The drawing under review shows one solid part. Ordinate dimensions are in mm from its lowest x, y, z. A direction names the side the tool comes from. Give positions to 0.01 mm unless a question says otherwise; leave off trailing zeros. Order: outer loops, then holes, each group sorted by start corner. A loop starts at its lowest first (then second) coordinate and runs counter-clockwise, first axis right, second up. Notation, with made-up numbers: (43, -33) -> (47, -33) arc R27 ccw to (47, 2) -> close; hole circle Ø3 at (-7, -5). An arc over 180 degrees is marked (long way). Return JSON: item names as keys, results as strings. Group by question number.
1) To check wall thickness, follow line 1 along Z through (x, y) = (31.75, 20.85); line 2 along Y through (x, z) = (27, 4.5); line 3 along X through (y, z) = (24.25, 3). State the ranges of each line that lie inside material, in increasing order.
2) For the marked faces 1, 2, 3 and 4, list the 3-axis set-ups (+Z, -Z, +X, -X, +Y, -Y) from which the entire face can be reached by the end or side of a thin tool; tool diameter is ignored.
3) Add section C-C (x = 66.5). Give the boundary of the cut face in (y, z).
4) Add section A-A (x = 133.35). Give the boundary of the cut face in (y, z), then the cut area to 3 significant figures.
5) Insertion check: P1, Ø3, axis at y = 9.525, z = 6.35, coming from the +X side; P2, Ø5, axis at x = 31.75, z = 6.35, coming from the -Y side; P3, Ø4, axis at y = 24, z = 7.5, coming from the -X side. Each pin has a flat end and moves straight along its axis. Give the tip position at first contact, or say it passes through.
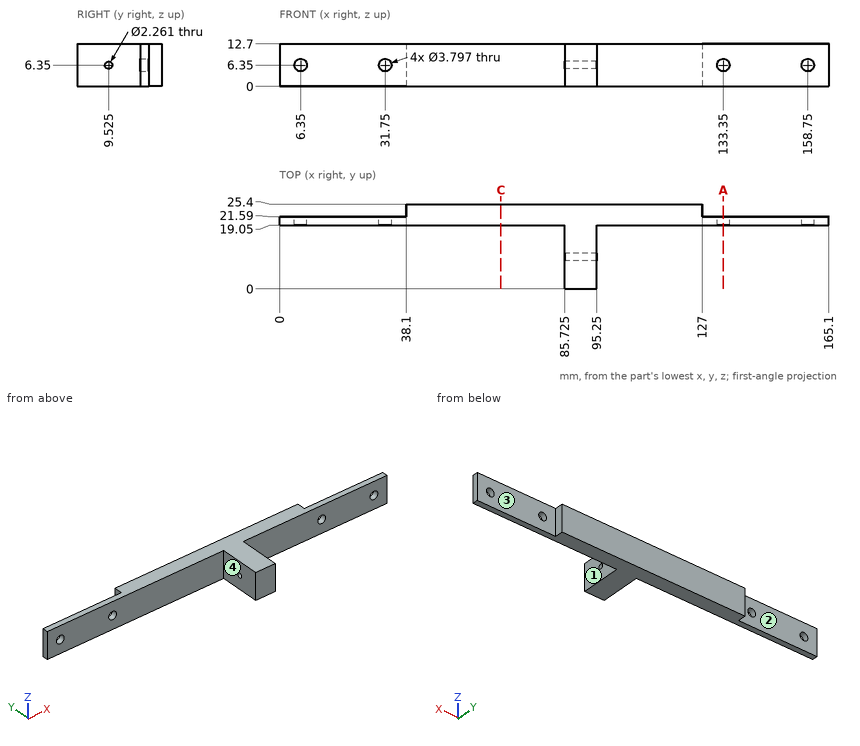
Evaluation:
{
 "1": {"line 1": "0 to 4.45, 8.25 to 12.7", "line 2": "19.05 to 21.59", "line 3": "38.1 to 127"},
 "2": {"face 1": "+Z, -Z, +X, -Y", "face 2": "+Z, -Z, -X, +Y", "face 3": "+Z, -Z, +X, +Y", "face 4": "+Z, -Z, -X, -Y"},
 "3": {"outline": "(19.05, 0) -> (25.4, 0) -> (25.4, 12.7) -> (19.05, 12.7) -> close"},
 "4": {"outline": "(19.05, 0) -> (21.59, 0) -> (21.59, 4.45) -> (19.05, 4.45) -> close; (19.05, 8.25) -> (21.59, 8.25) -> (21.59, 12.7) -> (19.05, 12.7) -> close", "area": "22.6 mm^2"},
 "5": {"P1": "x = 95.25", "P2": "y = 19.05", "P3": "x = 38.1"}
}
